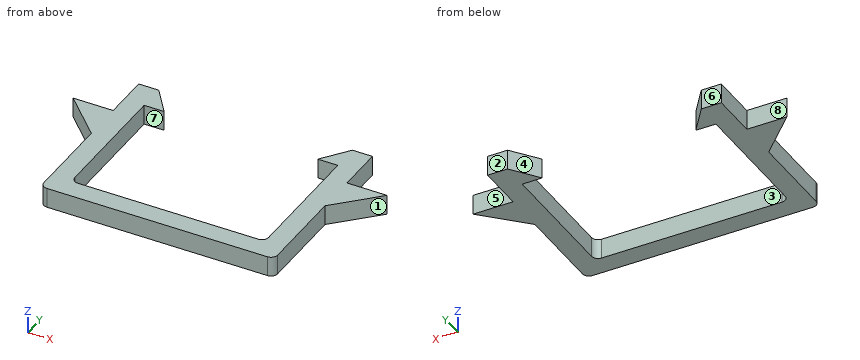
```python
from build123d import *

# Parameters (mm, degrees)
BOSS_EXTRUDE1_DEPTH = 1.5


with BuildPart() as part:
    # Sketch1 → Boss-Extrude1 (new, symmetric)
    with BuildSketch(Plane.XY):
        with BuildLine():
            Line((-13.5, 3), (13.5, 3))
            ThreePointArc((13.5, 3), (14.207106781, 3.292893219), (14.5, 4))
            Line((14.5, 4), (14.5, 23))
            Line((14.5, 23), (11.5, 23))
            Line((11.5, 23), (14.5, 27))
            Line((14.5, 27), (17.5, 27))
            Line((17.5, 27), (17.5, 20))
            Line((17.5, 20), (23.5, 20))
            Line((23.5, 20), (17.5, 14))
            Line((17.5, 14), (17.5, 1))
            ThreePointArc((17.5, 1), (17.207106781, 0.292893219), (16.5, 0))
            Line((16.5, 0), (-16.5, 0))
            ThreePointArc((-16.5, 0), (-17.207106781, 0.292893219), (-17.5, 1))
            Line((-17.5, 1), (-17.5, 14))
            Line((-17.5, 14), (-23.5, 20))
            Line((-23.5, 20), (-17.5, 20))
            Line((-17.5, 20), (-17.5, 27))
            Line((-17.5, 27), (-14.5, 27))
            Line((-14.5, 27), (-11.5, 23))
            Line((-11.5, 23), (-14.5, 23))
            Line((-14.5, 23), (-14.5, 4))
            ThreePointArc((-14.5, 4), (-14.207106781, 3.292893219), (-13.5, 3))
        make_face()
    extrude(amount=BOSS_EXTRUDE1_DEPTH, both=True)


solid = part.part
```
Here's how the part is built. I have some questions about the finished solid (model axes, mm). Face numbers are marked on the shaded views. A direction names the side the tool comes from. Coordinates: 2 decimals unless noted, no trailing zeros. Order: outer loops, then holes, each group sorted by start corner. A loop starts at its lowest first (then second) coordinate and runs counter-clockwise, first axis right, second up.
1) Which directions (+Z, -Z, +X, -X, +Y, -Y) give clear straight access to the entire face, cutting with the end or side of a thin tool? Please do the marked faces 4, 5, 6, 7 and 8.
2) Imagine slicing it at C-C on y = 5.5. List the corners of the cut face in (x, z) for me, and give its area (3 significant figures).
3) Will these pins go through, and if not, where does the flat tip stop? pin 1 (1.5 mm diameter, centred on y = 24.5, z = 0.5, fed in from +X); pin 2 (1.5 mm diameter, centred on x = -21, z = 0.5, fed in from +Y); pin 3 (1.5 mm diameter, centred on x = 12.5, z = -1, fed in from +Y).
4) Imagine slicing it at A-A on y = 16.5. List the corners of the cut face in (x, z) for me.
5) We'd pull the mould along X, two halves only. Please class the marked faces 1, 2 and 3: +X half, -X half, draft (parallel to the pull), parting line (faces both ways), or undercut.
6) I need wall thicknesses on line 1 (X direction, y = 5.25, z = -0.9); line 2 (Y direction, x = 4.5, z = 0.4); line 3 (X direction, y = 19, z = 0.7). Which ranges of each line are inside material? Lowest first, please.
7) Imagine slicing it at B-B on z = 0.35. List the corners of the cut face in (x, y) for me, and give its area (3 significant figures).
8) Imagine slicing it at D-D on x = 19. List the corners of the cut face in (y, z) for me.
Response values:
1. face 4: +Z, -Z, +Y
1. face 5: +Z, -Z, +X, +Y
1. face 6: +Z, -Z, +X, -X, +Y
1. face 7: +Z, -Z
1. face 8: +Z, -Z, -X, +Y
2. outline: (-17.5, -1.5) - (-14.5, -1.5) - (-14.5, 1.5) - (-17.5, 1.5) - close; (14.5, -1.5) - (17.5, -1.5) - (17.5, 1.5) - (14.5, 1.5) - close
2. area: 18.0 mm2
3. pin 1: stops at x = 17.5
3. pin 2: stops at y = 20
3. pin 3: stops at y = 25.33
4. outline: (-20, -1.5) - (-14.5, -1.5) - (-14.5, 1.5) - (-20, 1.5) - close; (14.5, -1.5) - (20, -1.5) - (20, 1.5) - (14.5, 1.5) - close
5. face 1: +X half
5. face 2: draft
5. face 3: undercut
6. line 1: x = -17.5 to -14.5, 14.5 to 17.5
6. line 2: y = 0 to 3
6. line 3: x = -22.5 to -14.5, 14.5 to 22.5
7. outline: (-23.5, 20) - (-17.5, 14) - (-17.5, 1) arc R1 ccw to (-16.5, 0) - (16.5, 0) arc R1 ccw to (17.5, 1) - (17.5, 14) - (23.5, 20) - (17.5, 20) - (17.5, 27) - (14.5, 27) - (11.5, 23) - (14.5, 23) - (14.5, 4) arc R1 cw to (13.5, 3) - (-13.5, 3) arc R1 cw to (-14.5, 4) - (-14.5, 23) - (-11.5, 23) - (-14.5, 27) - (-17.5, 27) - (-17.5, 20) - close
7. area: 297 mm2
8. outline: (15.5, -1.5) - (20, -1.5) - (20, 1.5) - (15.5, 1.5) - close
